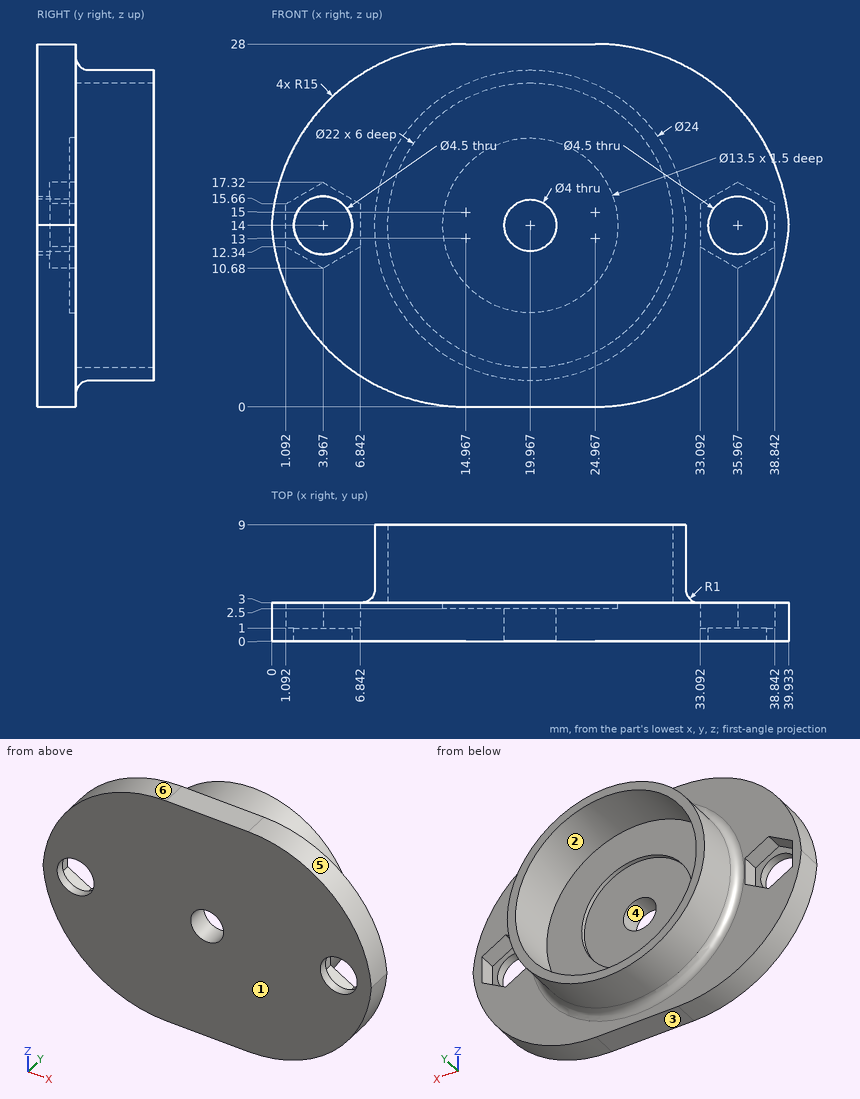
Drawing for the job (mm, zero at the part's lowest x, y, z). A direction names the side the tool comes from. Round coordinates to 2 decimals unless told otherwise and drop trailing zeros. One line per question, with ' | ' between items.
1. Mould opens along X. For the marked faces 3, 4, 5 and 6 say: pulls with the +X half, pulls with the -X half, needs draft (parallel to the pull), parting line crosses it, or undercut.
Working result:
face 3: needs draft | face 4: undercut | face 5: pulls with the +X half | face 6: pulls with the -X half
2. Probe L1, parallel to X at y = 2, z = 11 (1 decimal); L2, parallel to Z at x = 20, y = 4.5; L3, parallel to Y at x = 33, z = 17. List the from-to ranges inside material, lowest first. Write a range as from..to.
Working result:
L1: 0.5..3.4, 4.5..35.4, 36.5..39.4 | L2: 2..3, 25..26 | L3: 0..3
3. Pin check, flat tips, straight feed: pin 1 Ø1.5 at (y, z) = (4, 24.5) entering from +X; pin 2 Ø0.6 at (y, z) = (2, 13.5) entering from -X (1 decimal); pin 3 Ø4 at (y, z) = (8, 4) entering from -X. Stop position of each tip, or through.
Working result:
pin 1: x = 26.96 | pin 2: x = 0 | pin 3: x = 11.02
4. Which spindle directions (+Z, -Z, +X, -X, +Y, -Y) get a long thin tool onto all of the face, cutting with end or side? Do the marked faces 1 and 2. Say none if no direction does.
Working result:
face 1: +Z, -Z, +X, -X, -Y | face 2: +Y
